Here's how the part is built. I have some questions about the finished solid (model axes, mm). Face numbers are marked on the shaded views. A direction names the side the tool comes from. Coordinates: 2 decimals unless noted, no trailing zeros. Write each loop counter-clockwise with the first axis right and the second up, starting at its lowest first coordinate (ties: lowest second). Pieces come first, ordered by that corner, then holes.
Item 1: For the marked faces 1, 2 and 3, which set-ups out of +Z, -Z, +X, -X, +Y, -Y let a thin tool reach every point of the face, with its end or its side?
Item 2: If we section it at D-D (z = -0.75): Please give me the cut outline in (x, y), then the cut area to 3 significant figures.
Item 3: I'm going to push a flat-ended pin straight in: pin 1 Ø1.5 at (y, z) = (-0.5, -4.5) entering from -X. Where does the tip first touch, or does it pass through?
Item 4: If I drill on line 1 (Z direction, x = 0.6, y = 2.7); line 2 (X direction, y = 0.05, z = 3.5); line 3 (Y direction, x = 2.3, z = 0.5), over which ranges is the centre line in solid material (lowest first)?
Item 5: If we section it at A-A (y = 0): Please give me the cut outline in (x, z), then the cut area to 3 significant figures.
Item 6: If we section it at C-C (z = -4.5): Please give me the cut outline in (x, y).
from build123d import *

# Parameters (mm, degrees)
SKETCH1_R           = 2.55
BOSS_EXTRUDE1_DEPTH = 5
SKETCH2_R           = 3
BOSS_EXTRUDE2_DEPTH = 2
BOSS_EXTRUDE3_START = -7
SKETCH1_2_R         = 2.55
BOSS_EXTRUDE3_DEPTH = 5


with BuildPart() as part:
    # Sketch1 → Boss-Extrude1 (new body)
    with BuildSketch(Plane.XY):
        Circle(SKETCH1_R)
    extrude(amount=BOSS_EXTRUDE1_DEPTH)

    # Sketch2 → Boss-Extrude2 (add)
    with BuildSketch(Plane.XY):
        Circle(SKETCH2_R)
    extrude(amount=-BOSS_EXTRUDE2_DEPTH)

    # Sketch1<2> → Boss-Extrude3 (add)
    with BuildSketch(Plane.XY.offset(BOSS_EXTRUDE3_START)):
        Circle(SKETCH1_2_R)
    extrude(amount=BOSS_EXTRUDE3_DEPTH)


solid = part.part
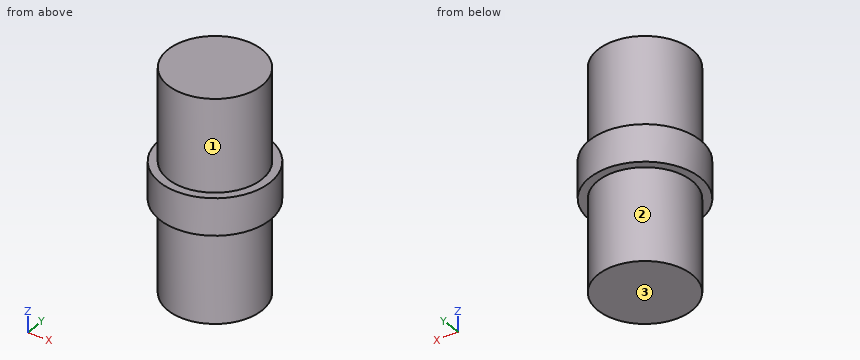
Answer list:
1. face 1: +Z
1. face 2: -Z
1. face 3: -Z, +X, -X, +Y, -Y
2. outline: circle Ø6 at (0, 0)
2. area: 28.3 mm2
3. pin 1: stops at x = -2.55
4. line 1: z = -2 to 0
4. line 2: x = -2.55 to 2.55
4. line 3: y = -1.1 to 1.1
5. outline: (-3, -2) - (-2.55, -2) - (-2.55, -7) - (2.55, -7) - (2.55, -2) - (3, -2) - (3, 0) - (2.55, 0) - (2.55, 5) - (-2.55, 5) - (-2.55, 0) - (-3, 0) - close
5. area: 63.0 mm2
6. outline: circle Ø5.1 at (0, 0)
